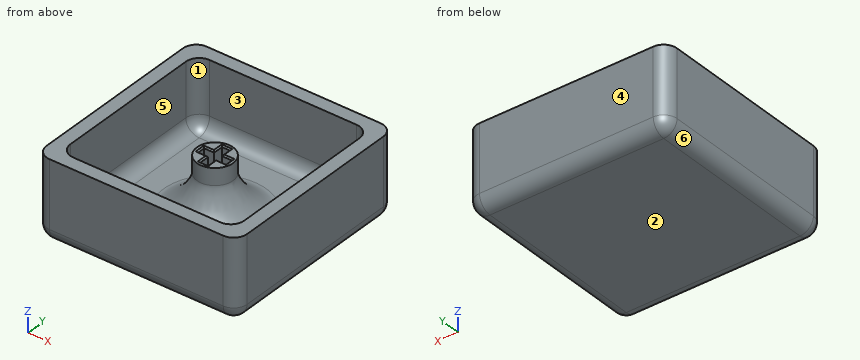
from build123d import *

# Parameters (mm, degrees)
EXTRUDE_1_DEPTH = 10
SKETCH_1_6_R    = 2.7
EXTRUDE_2_DEPTH = 8
EXTRUDE_START   = -2
EXTRUDE_3_DEPTH = 2
FILLET_1_R      = 2
CHAMFER_1_SIZE  = 0.2
FILLET_2_R      = 2
FILLET_3_SIZE   = 5
FILLET_3_SIZE_2 = 5.5


with BuildPart() as part:
    # Sketch 1 → Extrude 1 (new body)
    with BuildSketch(Plane.XY):
        with BuildLine():
            ThreePointArc((-15, 13), (-14.414213562, 14.414213562), (-13, 15))
            Line((-13, 15), (13, 15))
            ThreePointArc((13, 15), (14.414213562, 14.414213562), (15, 13))
            Line((15, 13), (15, -13))
            ThreePointArc((15, -13), (14.414213562, -14.414213562), (13, -15))
            Line((13, -15), (-13, -15))
            ThreePointArc((-13, -15), (-14.414213562, -14.414213562), (-15, -13))
            Line((-15, -13), (-15, 13))
        make_face()
        with BuildLine():
            ThreePointArc((-13, -11), (-12.414213562, -12.414213562), (-11, -13))
            Line((-11, -13), (11, -13))
            ThreePointArc((11, -13), (12.414213562, -12.414213562), (13, -11))
            Line((13, -11), (13, 11))
            ThreePointArc((13, 11), (12.414213562, 12.414213562), (11, 13))
            Line((11, 13), (-11, 13))
            ThreePointArc((-11, 13), (-12.414213562, 12.414213562), (-13, 11))
            Line((-13, 11), (-13, -11))
        make_face(mode=Mode.SUBTRACT)
    extrude(amount=EXTRUDE_1_DEPTH)



with BuildPart() as body_2:
    # Sketch 1_6 → Extrude 2 (new body)
    with BuildSketch(Plane.XY):
        Circle(SKETCH_1_6_R)
        Polygon((-2.085, -0.585), (-2.085, 0.585), (-0.585, 0.585), (-0.585, 2.085), (0.585, 2.085), (0.585, 0.585), (2.085, 0.585), (2.085, -0.585), (0.585, -0.585), (0.585, -2.085), (-0.585, -2.085), (-0.585, -0.585), align=None, mode=Mode.SUBTRACT)
    extrude(amount=EXTRUDE_2_DEPTH)


with BuildPart() as part_1:
    add(part.part)

    add(body_2.part)  # Extrude 3 merges body 2
    # Sketch 1_7 → Extrude 3 (add)
    with BuildSketch(Plane.XY.offset(EXTRUDE_START)):
        with BuildLine():
            Line((-13, 15), (13, 15))
            ThreePointArc((13, 15), (14.414213562, 14.414213562), (15, 13))
            Line((15, 13), (15, -13))
            ThreePointArc((15, -13), (14.414213562, -14.414213562), (13, -15))
            Line((13, -15), (-13, -15))
            ThreePointArc((-13, -15), (-14.414213562, -14.414213562), (-15, -13))
            Line((-15, -13), (-15, 13))
            ThreePointArc((-15, 13), (-14.414213562, 14.414213562), (-13, 15))
        make_face()
    extrude(amount=EXTRUDE_3_DEPTH)

    # Fillet 1
    fillet_1_edges = [part_1.edges().sort_by_distance(p)[0] for p in [
        (-14.414213562, -14.414213562, -2),
        (-15, 0, -2),
        (14.414213562, 14.414213562, -2),
        (14.414213562, -14.414213562, -2),
        (0, -15, -2),
        (-14.414213562, 14.414213562, -2),
        (0, 15, -2),
        (15, 0, -2),
    ]]
    fillet(fillet_1_edges, radius=FILLET_1_R)

    # Chamfer 1
    chamfer_1_edges = [part_1.edges().sort_by_distance(p)[0] for p in [
        (1.335, -0.585, 8),
        (0, -2.085, 8),
        (-0.585, -1.335, 8),
        (-1.335, -0.585, 8),
        (-2.085, 0, 8),
        (-0.585, 1.335, 8),
        (0, 2.085, 8),
        (0.585, 1.335, 8),
        (1.335, 0.585, 8),
        (2.085, 0, 8),
        (0.585, -1.335, 8),
        (-1.335, 0.585, 8),
    ]]
    chamfer(chamfer_1_edges, length=CHAMFER_1_SIZE)

    # Fillet 2
    fillet_2_edges = [part_1.edges().sort_by_distance(p)[0] for p in [
        (0, -13, 0),
        (12.414213562, -12.414213562, 0),
        (13, 0, 0),
        (12.414213562, 12.414213562, 0),
        (0, 13, 0),
        (-12.414213562, 12.414213562, 0),
        (-13, 0, 0),
        (-12.414213562, -12.414213562, 0),
    ]]
    fillet(fillet_2_edges, radius=FILLET_2_R)

    # Fillet 3
    # a fillet whose section is not a circle: 5.5, 5 mm, written as the material it adds along each edge
    with BuildSketch(Plane(origin=(0, 0, 0), x_dir=(1, 0, 0), z_dir=(0, -1, 0))) as fillet_3_piece_1:
        with BuildLine():
            Bezier((2.7 + FILLET_3_SIZE, 0), (2.7, 0), (2.7, FILLET_3_SIZE_2), weights=[1, 0.333333333, 1])
            Line((2.7, FILLET_3_SIZE_2), (2.7, 0))
            Line((2.7, 0), (2.7 + FILLET_3_SIZE, 0))
        make_face()
    revolve(axis=Axis((0, 0, 0), (0, 0, 1)))


solid = part_1.part
Source: CAD feature listing. Evaluate the final solid. Frame: model axes, mm. Face numbers are marked on the shaded views. A direction names the side the tool comes from. Give positions to 0.01 mm unless a question says otherwise; leave off trailing zeros. Loops run counter-clockwise (first coordinate to the right, second up) from the corner with the lowest first, then second, coordinate; pieces in that order, holes last. Notation, with made-up numbers: (54.25, 13.25) -> (86.25, 13.25) arc R23 cw to (86.25, 43.25) -> close; hole circle Ø7 at (83.25, 11.5). An arc over 180 degrees is marked (long way). Use a Markdown table: item, result. Add a question column.
1) Section query A-A, the plane z = 9.25. Return the cut outline in (x, y), then the cut area to 3 significant figures.
2) Pull-direction query (Y, two-part tool) for the marked faces 3, 4, 5 and 6; classes: +Y half, -Y half, draft (parallel to the pull), parting line (faces both ways), or undercut.
3) Section query D-D, the plane z = -1. Return the cut outline in (x, y), then the cut area to 3 significant figures.
4) Reachability of the marked faces 1 and 2 from +Z, -Z, +X, -X, +Y, -Y: full face, straight path, thin tool, end or side. Return the list, or none.
5) Line query: line 1 along X through (y, z) = (-2.5, 8.75); line 2 along X through (y, z) = (-0.5, 3.25) (3 decimals). Output: solid intervals per line, ascending. Write a range as [from, to].
6) Section query B-B, the plane x = -9.25. Return the cut outline in (y, z).
7) First-contact query: pin 1 (6 mm diameter, centred on x = 1, y = 0.5, fed in from +Z); pin 2 (8 mm diameter, centred on x = -8, y = 5.5, fed in from +Z). Flat tips, straight axial feed; report the tip coordinate or a pass-through.
Numbers:
| question | item | result |
|---|---|---|
| 1 | outline | (-15, -13) arc R2 ccw to (-13, -15) -> (13, -15) arc R2 ccw to (15, -13) -> (15, 13) arc R2 ccw to (13, 15) -> (-13, 15) arc R2 ccw to (-15, 13) -> close; hole (-13, -11) arc R2 ccw to (-11, -13) -> (11, -13) arc R2 ccw to (13, -11) -> (13, 11) arc R2 ccw to (11, 13) -> (-11, 13) arc R2 ccw to (-13, 11) -> close |
| 1 | area | 224 mm2 |
| 2 | face 3 | undercut |
| 2 | face 4 | +Y half |
| 2 | face 5 | undercut |
| 2 | face 6 | draft |
| 3 | outline | (-14.73, -13) arc R1.73 ccw to (-13, -14.73) -> (13, -14.73) arc R1.73 ccw to (14.73, -13) -> (14.73, 13) arc R1.73 ccw to (13, 14.73) -> (-13, 14.73) arc R1.73 ccw to (-14.73, 13) -> close |
| 3 | area | 866 mm2 |
| 4 | face 1 | +Z |
| 4 | face 2 | -Z, +X, -X, +Y, -Y |
| 5 | line 1 | x = [-15, -13], [13, 15] |
| 5 | line 2 | x = [-15, -13], [-3.602, -2.085], [2.085, 3.602], [13, 15] |
| 6 | outline | (-15, 0) arc R2 ccw to (-13, -2) -> (13, -2) arc R2 ccw to (15, 0) -> (15, 10) -> (13, 10) -> (13, 2) arc R2 cw to (11, 0) -> (-11, 0) arc R2 cw to (-13, 2) -> (-13, 10) -> (-15, 10) -> close |
| 7 | pin 1 | stops at z = 8 |
| 7 | pin 2 | stops at z = 0.99 |
